Geometry check sheet. Reference: the model listing, model coordinates, mm. A direction names the side the tool comes from. Coordinates: 2 decimals unless noted, no trailing zeros. Loops run counter-clockwise (first coordinate to the right, second up) from the corner with the lowest first, then second, coordinate; pieces in that order, holes last.
from build123d import *

# Parameters (mm, degrees)
F0_R     = 12.5
F1_DEPTH = 5.28
F2_R     = 8.65
F3_DEPTH = 4.32
F4_R     = 5
F5_DEPTH = 4.32
F6_W     = 4.5
F6_H     = 0.3
F8_R     = 2.4
F9_DEPTH = 25


with BuildPart() as f1:
    # F0 (on Front) → F1 (new body)
    with BuildSketch(Plane.XZ):
        Circle(F0_R)
    extrude(amount=F1_DEPTH)

    # F2 (on face) → F3 (join)
    with BuildSketch(Plane(origin=(0, 0, 0), x_dir=(-1, 0, 0), z_dir=(0, 1, 0))):
        Circle(F2_R)
    extrude(amount=F3_DEPTH)

    # F4 (on face) → F5 (cut)
    with BuildSketch(Plane.XZ.offset(5.28)):
        Circle(F4_R)
    extrude(amount=-F5_DEPTH, mode=Mode.SUBTRACT)

    # F6 (on Right) → F7 (revolve, cut)
    with BuildSketch(Plane.YZ):
        with Locations((-2.64, 12.35)):
            Rectangle(F6_W, F6_H)
    revolve(axis=Axis((0, 0, 0), (0, 1, 0)), mode=Mode.SUBTRACT)

    # F8 (on face) → F9 (cut)
    with BuildSketch(Plane.XZ.offset(0.96)):
        Circle(F8_R)
    extrude(amount=-F9_DEPTH, mode=Mode.SUBTRACT)


solid = f1.part
(1) Sectioned sample at C-C on y = -4.5. Record the cut outline in (x, z).
Findings:
outline: circle Ø24.4 at (0, 0); hole circle Ø10 at (0, 0)
(2) Sectioned sample at B-B on x = 0. Record the cut outline in (y, z), and give its area (3 significant figures).
Findings:
outline: (-5.28, -12.5) - (-4.89, -12.5) - (-4.89, -12.2) - (-0.39, -12.2) - (-0.39, -12.5) - (0, -12.5) - (0, -8.65) - (4.32, -8.65) - (4.32, -2.4) - (-0.96, -2.4) - (-0.96, -5) - (-5.28, -5) - close; (-5.28, 5) - (-0.96, 5) - (-0.96, 2.4) - (4.32, 2.4) - (4.32, 8.65) - (0, 8.65) - (0, 12.5) - (-0.39, 12.5) - (-0.39, 12.2) - (-4.89, 12.2) - (-4.89, 12.5) - (-5.28, 12.5) - close
area: 135 mm2
(3) Scan lines: L1, parallel to Z at x = 0, y = 1.5; L2, parallel to Y at x = 8, z = -7; L3, parallel to Y at x = -1, z = -4.5. Record each from-to range of solid material in increasing order.
Findings:
L1: z = -8.65 to -2.4, 2.4 to 8.65
L2: y = -5.28 to 0
L3: y = -0.96 to 4.32
(4) Sectioned sample at A-A on z = 0. Record the cut outline in (x, y).
Findings:
outline: (-12.5, -5.28) - (-5, -5.28) - (-5, -0.96) - (-2.4, -0.96) - (-2.4, 4.32) - (-8.65, 4.32) - (-8.65, 0) - (-12.5, 0) - (-12.5, -0.39) - (-12.2, -0.39) - (-12.2, -4.89) - (-12.5, -4.89) - close; (2.4, -0.96) - (5, -0.96) - (5, -5.28) - (12.5, -5.28) - (12.5, -4.89) - (12.2, -4.89) - (12.2, -0.39) - (12.5, -0.39) - (12.5, 0) - (8.65, 0) - (8.65, 4.32) - (2.4, 4.32) - close
(5) Gauge pin test, flat ends, axial feed: pin 1 Ø2 at (y, z) = (-3.5, 10) entering from -X; pin 2 Ø3 at (x, z) = (0, -2) entering from -Y; pin 3 Ø1 at (x, y) = (8, 1) entering from -Z. Record the tip position at first contact, or that the pin passes through.
Findings:
pin 1: stops at x = -8.24
pin 2: stops at y = -0.96
pin 3: stops at z = -4.31
(6) Draft check along Y on faces 4 (the flat face through (-0.2, -5.28, -5.4)), 5 (the cylindrical face through (0.54, -2.61, -12.19)), 6 (the cylindrical face through (11.923, -5.082, 3.755)). Enter one of: +Y half, -Y half, draft (parallel to the pull), parting line (faces both ways), or undercut.
Findings:
face 4: -Y half
face 5: undercut
face 6: draft
(7) Access from +Z, -Z, +X, -X, +Y, -Y to the whole of each face (thin tool, end or side, straight path). Record for faces 1 (the cylindrical face through (-8.25, 2.13, 2.6)), 2 (the cylindrical face through (11.923, -0.192, 3.755)), 3 (the flat face through (-1.2, -0.96, 2.3)).
Findings:
face 1: +Y
face 2: +Y, -Y
face 3: -Y
(8) Sectioned sample at D-D on x = 10.5. Record the cut outline in (y, z), and give its area (3 significant figures).
Findings:
outline: (-5.28, -6.78) - (-4.89, -6.78) - (-4.89, -6.21) - (-0.39, -6.21) - (-0.39, -6.78) - (0, -6.78) - (0, 6.78) - (-0.39, 6.78) - (-0.39, 6.21) - (-4.89, 6.21) - (-4.89, 6.78) - (-5.28, 6.78) - close
area: 66.5 mm2
